from build123d import *

# Parameters (mm, degrees)
MAIN_FRAME_PROFILE_R        = 10.668
CROSS_BAR_BOTTOM_PROFILE_R  = 6.35
SWIVEL_CONNECTION_PROFILE_R = 6.35
SWIVEL_OUTER_PROFILE_R      = 12.7


with BuildPart() as part:
    # Main Frame: sweep along a curve in space
    with BuildLine() as main_frame_path:
        Line((190.5, 0, 19.05), (190.5, 0, 208.874106245))
        ThreePointArc((190.5, 0, 208.874106245), (190.5, -0.869202084, 222.135567375), (190.5, -3.461936049, 235.170121228))
        Line((190.5, -3.461936049, 235.170121228), (190.5, -96.590179262, 582.729456518))
        ThreePointArc((186.008430573, -99.081814666, 628.564887795), (189.362259809, -100.245120407, 605.624792126), (190.5, -96.590179262, 582.729456518))
        Line((142.782679241, -64.080286866, 849.555836961), (186.008430573, -99.081814666, 628.564887795))
        ThreePointArc((80.435511173, -56.030942434, 900.377397559), (120.854542376, -58.303150976, 886.031237436), (142.782679241, -64.080286866, 849.555836961))
        Line((0, -56.030942434, 900.377397559), (80.435511173, -56.030942434, 900.377397559))
    # Main Frame profile (on start of the path) → Main Frame (sweep)
    with BuildSketch(Plane(origin=(190.5, 0, 19.05), x_dir=(0, 1, 0), z_dir=(0, 0, 1))):
        Circle(MAIN_FRAME_PROFILE_R)
    main_frame = sweep(path=main_frame_path.line)

    # Cross Bar Bottom: sweep along a curve in space
    with BuildLine() as cross_bar_bottom_path:
        Line((190.5, 0, 38.1), (0, 0, 38.1))
    # Cross Bar Bottom profile (on start of the path) → Cross Bar Bottom (sweep)
    with BuildSketch(Plane(origin=(190.5, 0, 38.1), x_dir=(0, -1, 0), z_dir=(-1, 0, 0))):
        Circle(CROSS_BAR_BOTTOM_PROFILE_R)
    cross_bar_bottom = sweep(path=cross_bar_bottom_path.line)

    # Swivel Connection: sweep along a curve in space
    with BuildLine() as swivel_connection_path:
        Line((190.5, 0, 0), (190.5, 0, 19.05))
    # Swivel Connection profile (on start of the path) → Swivel Connection (sweep)
    with BuildSketch(Plane(origin=(190.5, 0, 0), x_dir=(0, 1, 0), z_dir=(0, 0, 1))):
        Circle(SWIVEL_CONNECTION_PROFILE_R)
    swivel_connection = sweep(path=swivel_connection_path.line)

    # Swivel Outer: sweep along a curve in space
    with BuildLine() as swivel_outer_path:
        Line((201.6125, 0, 0), (177.8, 0, 0))
    # Swivel Outer profile (on start of the path) → Swivel Outer (sweep)
    with BuildSketch(Plane(origin=(201.6125, 0, 0), x_dir=(0, -1, 0), z_dir=(-1, 0, 0))):
        Circle(SWIVEL_OUTER_PROFILE_R)
    swivel_outer = sweep(path=swivel_outer_path.line)

    # Mirror1: Main Frame, Cross Bar Bottom, Swivel Connection, Swivel Outer across plane
    add(main_frame.mirror(Plane(origin=(0, 0, 0), x_dir=(0, 0, 1), z_dir=(1, 0, 0))))
    add(cross_bar_bottom.mirror(Plane(origin=(0, 0, 0), x_dir=(0, 0, 1), z_dir=(1, 0, 0))))
    add(swivel_connection.mirror(Plane(origin=(0, 0, 0), x_dir=(0, 0, 1), z_dir=(1, 0, 0))))
    add(swivel_outer.mirror(Plane(origin=(0, 0, 0), x_dir=(0, 0, 1), z_dir=(1, 0, 0))))


solid = part.part
Read the model definition and answer for the solid it produces. Units are mm, in the model's axes. A direction names the side the tool comes from. Coordinates: 2 decimals unless noted, no trailing zeros. Loops run counter-clockwise (first coordinate to the right, second up) from the corner with the lowest first, then second, coordinate; pieces in that order, holes last. Notation, with made-up numbers: (29, 86) - (60, 86) arc R16 cw to (60, 95) - close; hole circle Ø10 at (52, -25.5). An arc over 180 degrees is marked (long way). Answer in a Markdown table with one row per item.
Q1. Straight lines are drawn through the part: line 1 along X through (y, z) = (-0.5, 138); line 2 along Y through (x, z) = (181, 669.5); line 3 along X through (y, z) = (-90, 704). For each, find the intervals that lie inside material, in ascending order. Write a range as [from, to].
Here are the results:
| item | result |
|---|---|
| line 1 | x = [-201.16, -179.84], [179.84, 201.16] |
| line 2 | y = [-103.07, -82.31] |
| line 3 | x = [-181.82, -160.86], [160.86, 181.82] |
Q2. Find section A-A on z = 0. Write down the section's boundary in (x, y).
Here are the results:
| item | result |
|---|---|
| outline | (-201.61, -12.7) - (-177.8, -12.7) - (-177.8, 12.7) - (-201.61, 12.7) - close; (177.8, -12.7) - (201.61, -12.7) - (201.61, 12.7) - (177.8, 12.7) - close |
Q3. Given P1, Ø12, axis at y = -47.5, z = 347.5, coming from the -X side; P2, Ø1, axis at y = -80.5, z = 782, coming from the -X side; P3, Ø12, axis at x = -111, y = -66, coming from the +Z side, each flat-ended and moving along its own axis, determine where each tip first touches the part or whether it passes through.
Here are the results:
| item | result |
|---|---|
| P1 | stops at x = -198.12 |
| P2 | stops at x = -165.7 |
| P3 | stops at z = 904.97 |
Q4. The mould has two halves that part along X. Classify faces 3 (the cylindrical face through (173.574, -76.572, 741.707)), 4 (the flat face through (201.612, 0, 0)), 5 (the flat face through (-201.612, 0, 0)): pulls with the +X half, pulls with the -X half, needs draft (parallel to the pull), parting line crosses it, or undercut.
Here are the results:
| item | result |
|---|---|
| face 3 | undercut |
| face 4 | pulls with the +X half |
| face 5 | pulls with the -X half |
Q5. For faces 1 (the flat face through (-177.8, 0, 0)), 2 (the cylindrical face through (179.923, -1.389, 115.291)), determine the directions among +Z, -Z, +X, -X, +Y, -Y from which every point of the face is accessible in a straight line to the end or side of a thin tool.
Here are the results:
| item | result |
|---|---|
| face 1 | -Z, +Y, -Y |
| face 2 | none |
Q6. Find section B-B on x = 41. Write down the section's boundary in (y, z).
Here are the results:
| item | result |
|---|---|
| outline | circle Ø21.34 at (-56.03, 900.38); circle Ø12.7 at (0, 38.1) |
